Geometry check sheet. Reference: the model listing, model coordinates, mm. Round coordinates to 2 decimals unless told otherwise and drop trailing zeros. Write each loop counter-clockwise with the first axis right and the second up, starting at its lowest first coordinate (ties: lowest second). Pieces come first, ordered by that corner, then holes.
Item 1: Cross-section at C-C (x = -177). Enter the section's corners in (y, z).
Item 2: Cross-section at A-A (z = -399). Enter the section's corners in (x, y), then the cut area to 3 significant figures.
Item 3: Depth check by flat-ended pin: P1, Ø1, axis at x = -112, y = 1.5, coming from the -Z side; P2, Ø1, axis at x = -1012, y = 0.5, coming from the -Z side. Enter the tip coordinate at first touch or a pass-through.
Item 4: Scan lines: probe 1 along Z at (x, y) = (-383, 0.55); probe 2 along Z at (x, y) = (-87, 0.55). Record each from-to range of solid material in increasing order.
Item 5: Cross-section at B-B (y = 1.35). Enter the section's corners in (x, z), then the cut area to 3 significant figures.
Autodesk Inventor part; units mm, degrees
ref_plane "YZ Plane" through (0, 0, 0) normal (1, 0, 0) x (0, 1, 0)
ref_plane "XZ Plane" through (0, 0, 0) normal (0, 1, 0) x (-1, 0, 0)
ref_plane "XY Plane" through (0, 0, 0) normal (0, 0, 1) x (1, 0, 0)
sketch "Sketch1" plane through (0, 0, 0) normal (0, 1, 0) x (-1, 0, 0)
  line L0 (0, 0) -> (1020, 0)
  line L1 (0, -425.23) -> (0, 0)
  line L2 (1020, 0) -> (1020, -425.23)
  line L3 (1020, -425.23) -> (0, -425.23)
  dimension "d0" = 425.23
  dimension "d1" = 1020
extrude "Plate1" add sketch "Sketch1" along normal blind 2
sketch "Sketch2" plane through (0, 0, 0) normal (0, -1, 0) x (1, 0, 0)
  line L0 (0, -425.2298) -> (-1007.836, -30)
  line L1 (-996, -30) -> (-1014, -30)
  arc A0 (-1020, -24) -> (-1014, -30) centre (-1014, -24) ccw
  line L2 (0, -425.23) -> (-1020, -425.23)
  line L3 (0, 0) -> (0, -425.23)
  line L4 (-1020, 0) -> (0, 0)
  line L5 (-1020, -425.23) -> (-1020, 0)
extrude "Extrusion1" cut sketch "Sketch2" against normal through all contours L2 L5 A0 L1 L0
equation "\"d2\" = Thickness"
equation "\"BendRadius\" = Thickness"
equation "\"BendReliefWidth\" = Thickness"
equation "\"BendReliefDepth\" = 0.5 * Thickness"
equation "\"CornerReliefSize\" = 4 * Thickness"
equation "\"MinimumRemnant\" = 2 * Thickness"
equation "\"TransitionRadius\" = BendRadius"
equation "\"JacobiRadiusSize\" = BendRadius"
equation "\"GapSize\" = Thickness"
properties part number "taringle"
Resolved:
1. outline: (0, -355.82) - (2, -355.82) - (2, 0) - (0, 0) - close
2. outline: (-66.89, 0) - (0, 0) - (0, 2) - (-66.89, 2) - close
2. area: 134 mm2
3. P1: stops at z = -381.5
3. P2: stops at z = -30
4. probe 1: z = -275.03 to 0
4. probe 2: z = -391.11 to 0
5. outline: (-1020, -24) arc R6 ccw to (-1014, -30) - (-1007.84, -30) - (0, -425.23) - (0, 0) - (-1020, 0) - close
5. area: 230,000 mm2
